The model under review builds one solid part; all positions refer to its coordinate system, in mm. Give positions to 0.01 mm unless a question says otherwise; leave off trailing zeros. Order: outer loops, then holes, each group sorted by start corner. A loop starts at its lowest first (then second) coordinate and runs counter-clockwise, first axis right, second up.
```python
from build123d import *

# Parameters (mm, degrees)
MODEL_R                  = 1.5
MODEL_W                  = 90
MODEL_H                  = 40
RESSALTO_EXTRUS_O1_DEPTH = 6


with BuildPart() as part:
    # Model → Ressalto-extrusão1 (new body)
    with BuildSketch(Plane.XY):
        Polygon((36.5, -62), (36.5, -70), (40, -70), (40, -75), (50, -75), (50, -70), (140, -70), (140, -75), (150, -75), (150, -70), (153.5, -70), (153.5, -62), (151.5, -62), (151.5, -57), (158.5, -57), (158.5, -62), (156.5, -62), (156.5, -70), (160, -70), (160, -75), (170, -75), (170, -70), (190, -70), (190, 0), (170, 0), (170, 5), (160, 5), (160, 0), (156.5, 0), (156.5, -8), (158.5, -8), (158.5, -13), (151.5, -13), (151.5, -8), (153.5, -8), (153.5, 0), (150, 0), (150, 5), (140, 5), (140, 0), (50, 0), (50, 5), (40, 5), (40, 0), (36.5, 0), (36.5, -8), (38.5, -8), (38.5, -13), (31.5, -13), (31.5, -8), (33.5, -8), (33.5, 0), (30, 0), (30, 5), (20, 5), (20, 0), (0, 0), (0, -70), (20, -70), (20, -75), (30, -75), (30, -70), (33.5, -70), (33.5, -62), (31.5, -62), (31.5, -57), (38.5, -57), (38.5, -62), align=None)
        with Locations((30, -32)):
            Circle(MODEL_R, mode=Mode.SUBTRACT)
        with Locations((150, -50)):
            Circle(MODEL_R, mode=Mode.SUBTRACT)
        with Locations((40, -20)):
            Circle(MODEL_R, mode=Mode.SUBTRACT)
        with Locations((150, -20)):
            Circle(MODEL_R, mode=Mode.SUBTRACT)
        with Locations((40, -50)):
            Circle(MODEL_R, mode=Mode.SUBTRACT)
        with Locations((160, -32)):
            Circle(MODEL_R, mode=Mode.SUBTRACT)
        with Locations((95, -30)):
            Rectangle(MODEL_W, MODEL_H, mode=Mode.SUBTRACT)
    extrude(amount=RESSALTO_EXTRUS_O1_DEPTH)


solid = part.part
```
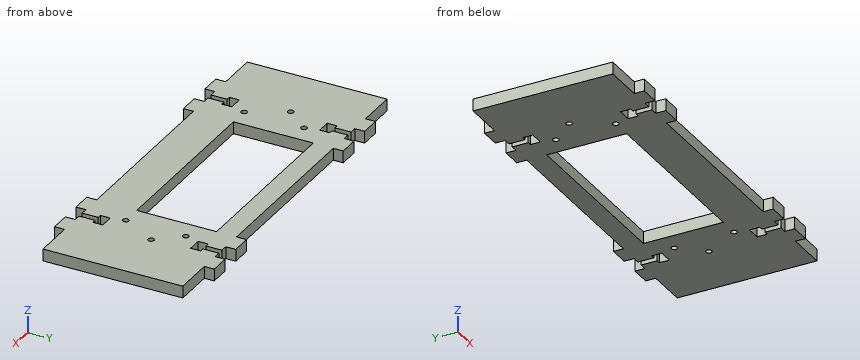
Item 1: For line 1 (X direction, y = -7, z = 1.05); line 2 (Y direction, x = 78, z = 3); line 3 (X direction, y = -29, z = 1.4), list the stretches that pass through material, from the lowest coordinate up.
Values found:
line 1: x = 0 to 33.5, 36.5 to 153.5, 156.5 to 190
line 2: y = -70 to -50, -10 to 0
line 3: x = 0 to 50, 140 to 190
Item 2: Take a section at C-C (z = 1.6). Give the number of separate pieces and of enclosed holes in the cut face, and give its area (3 significant figures).
Values found:
separate pieces: 1
enclosed holes: 7
area: 9,820 mm2
Item 3: Take a section at A-A (y = -45.5). Give the boundary of the cut face in (x, z), and give its area (3 significant figures).
Values found:
outline: (0, 0) - (50, 0) - (50, 6) - (0, 6) - close; (140, 0) - (190, 0) - (190, 6) - (140, 6) - close
area: 600 mm2
Item 4: Clearance check with flat-ended pins moving along their axes: pin 1 Ø1.5 at (y, z) = (3.5, 3.5) entering from -X; pin 2 Ø2.5 at (x, y) = (160, -32) entering from +Z; pin 3 Ø2.5 at (y, z) = (3, 2) entering from +X; pin 4 Ø1 at (y, z) = (-4.5, 2.5) entering from -X. State where each tip first meets the part, or that it passes through.
Values found:
pin 1: stops at x = 20
pin 2: passes through
pin 3: stops at x = 170
pin 4: stops at x = 0
Item 5: Take a section at B-B (y = -3.5). Give the boundary of the cut face in (x, z), and give its area (3 significant figures).
Values found:
outline: (0, 0) - (33.5, 0) - (33.5, 6) - (0, 6) - close; (36.5, 0) - (153.5, 0) - (153.5, 6) - (36.5, 6) - close; (156.5, 0) - (190, 0) - (190, 6) - (156.5, 6) - close
area: 1,100 mm2
